Check sheet for the drawn part. Datum: minimum x, y, z corner. Units: mm. A direction names the side the tool comes from. Coordinates: 2 decimals unless noted, no trailing zeros. Order: outer loops, then holes, each group sorted by start corner. A loop starts at its lowest first (then second) coordinate and runs counter-clockwise, first axis right, second up. Notation, with made-up numbers: (39.25, 21.25) - (54.25, 21.25) arc R15 cw to (54.25, 28.25) - close; hole circle Ø6 at (55, 23.25). An arc over 180 degrees is marked (long way). Return JSON: item names as keys, results as strings. Group by question number.
Item 1: Draft check along Y on the marked faces 1, 2 and 3. Enter one of: pulls with the +Y half, pulls with the -Y half, needs draft (parallel to the pull), parting line crosses it, or undercut.
Item 2: Section check B-B on y = 20.5. Enter the section's corners in (x, z), then the cut area to 3 significant figures.
Item 3: Gauge pin test, flat end, axial feed: pin 1 (1.5 mm diameter, centred on x = 26.5, y = 3, fed in from -Z). Record the tip position at first contact, or that the pin passes through.
Item 4: Section check A-A on z = 15. Enter the section's corners in (x, y), then the cut area to 3 significant figures.
Item 5: Scan lines: probe 1 along Y at (x, z) = (15, 27); probe 2 along Y at (x, z) = (6, 15); probe 3 along Z at (x, y) = (27.5, 14.5). Record each from-to range of solid material in increasing order.
Item 6: Section check C-C on y = 12.5. Enter the section's corners in (x, z).
Item 7: Tool access check on the marked faces 4 and 5. Record the directions out of +Z, -Z, +X, -X, +Y, -Y that give a thin tool (end or side, any length) a straight path to the whole face; none if there is none.
Item 8: Section check D-D on x = 6.5. Enter the section's corners in (y, z), then the cut area to 3 significant figures.
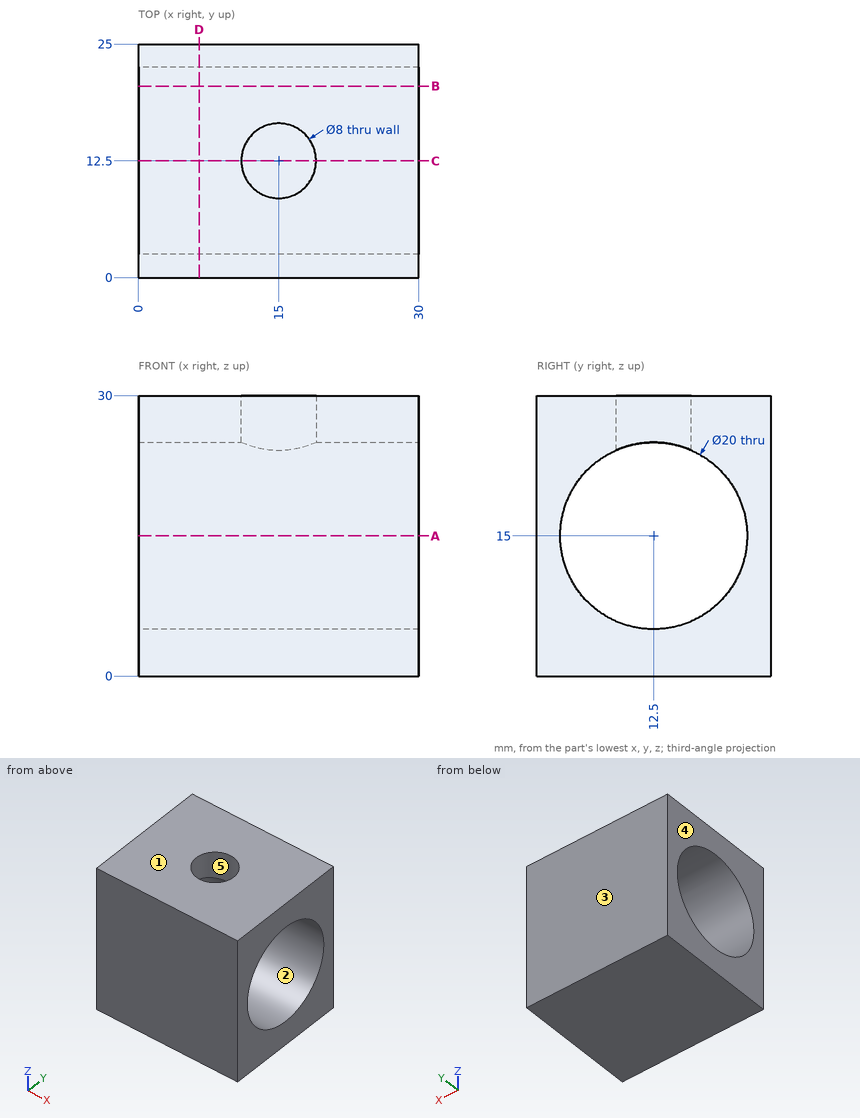
Computed:
{
 "1": {"face 1": "needs draft", "face 2": "undercut", "face 3": "pulls with the +Y half"},
 "2": {"outline": "(0, 0) - (30, 0) - (30, 9) - (0, 9) - close; (0, 21) - (30, 21) - (30, 30) - (0, 30) - close", "area": "540 mm²"},
 "3": {"pin 1": "stops at z = 0"},
 "4": {"outline": "(0, 0) - (30, 0) - (30, 2.5) - (0, 2.5) - close; (0, 22.5) - (30, 22.5) - (30, 25) - (0, 25) - close", "area": "150 mm²"},
 "5": {"probe 1": "y = 0 to 8.5, 16.5 to 25", "probe 2": "y = 0 to 2.5, 22.5 to 25", "probe 3": "z = 0 to 5.2, 24.8 to 30"},
 "6": {"outline": "(0, 0) - (30, 0) - (30, 5) - (0, 5) - close; (0, 25) - (11, 25) - (11, 30) - (0, 30) - close; (19, 25) - (30, 25) - (30, 30) - (19, 30) - close"},
 "7": {"face 4": "+Z, -Z, -X, +Y, -Y", "face 5": "+Z"},
 "8": {"outline": "(0, 0) - (25, 0) - (25, 30) - (0, 30) - close; hole circle Ø20 at (12.5, 15)", "area": "436 mm²"}
}
